```python
from build123d import *

# Parameters (mm, degrees)
F0_R      = 127
F1_DEPTH  = 254
F3_DEPTH  = 254
F4_DEPTH  = 25.4
F5_R      = 49.5787296889
F6_DEPTH  = 210.82
F7_R      = 54.002568176
F8_DEPTH  = 254
F9_R      = 52.4914497997
F10_DEPTH = 254


with BuildPart() as f1:
    # F0 (on Top) → F1 (new body)
    with BuildSketch(Plane.XY):
        Circle(F0_R)
    extrude(amount=F1_DEPTH)

    # F2 (on face) → F3 (join)
    with BuildSketch(Plane.XY.offset(254)):
        with BuildLine():
            Line((559.1962337494, 39.9803072214), (126.6766473602, 9.056876591))
            ThreePointArc((126.6766473602, 9.056876591), (126.9191360961, 4.5313234964), (127, 0))
            ThreePointArc((127, 0), (124.2007035095, -26.5176403124), (115.9262165711, -51.8662926332))
            Line((115.9262165711, -51.8662926332), (503.8578976831, -62.8307757108))
            Line((503.8578976831, -62.8307757108), (513.781719797, -288.9111098311))
            Line((513.781719797, -288.9111098311), (573.5178616361, -286.2889850555))
            Line((573.5178616361, -286.2889850555), (559.1962337494, 39.9803072214))
        make_face()
    extrude(amount=-F3_DEPTH)

    # F4 (add): a face of the model
    f4_faces = [f1.faces().sort_by_distance(p)[0] for p in [
        (309.8920571271, -57.348534172, 127),
    ]]
    extrude(f4_faces, amount=F4_DEPTH)

    # F5 (on face) → F6 (cut)
    with BuildSketch(Plane(origin=(-2.08986034, -73.9408350817, 0), x_dir=(0.9996008136, -0.0282526711, 0), z_dir=(-0.0282526711, -0.9996008136, 0))):
        with Locations((185.5181306601, 163.3890718222)):
            Circle(F5_R)
    extrude(amount=-F6_DEPTH, mode=Mode.SUBTRACT)

    # F7 (on face) → F8 (cut)
    with BuildSketch(Plane(origin=(-2.08986034, -73.9408350817, 0), x_dir=(0.9996008136, -0.0282526711, 0), z_dir=(-0.0282526711, -0.9996008136, 0))):
        with Locations((322.3161399364, 168.2878434658)):
            Circle(F7_R)
    extrude(amount=-F8_DEPTH, mode=Mode.SUBTRACT)

    # F9 (on face) → F10 (cut)
    with BuildSketch(Plane(origin=(-2.08986034, -73.9408350817, 0), x_dir=(0.9996008136, -0.0282526711, 0), z_dir=(-0.0282526711, -0.9996008136, 0))):
        with Locations((390.9286558628, 74.9529749155)):
            Circle(F9_R)
    extrude(amount=-F10_DEPTH, mode=Mode.SUBTRACT)


solid = f1.part
```
Design review of the part built by this model. Coordinates are the model's own, in mm. A direction names the side the tool comes from. Coordinates: 2 decimals unless noted, no trailing zeros. Loops run counter-clockwise (first coordinate to the right, second up) from the corner with the lowest first, then second, coordinate; pieces in that order, holes last. Notation, with made-up numbers: M 54.5,3.25 L 103.5,3.25 A19 cw 103.5,33.25 Z; hole C -35,-1 d6. An arc over 180 degrees is marked long. One line per question, with ' | ' between items.
(1) Draft analysis for pull direction X (two halves, no side actions). For faces 1 (the face through (230.49, -32.44, 144.4)), 2 (the face through (221, -33, 0)), 3 (the face through (543.23, -287.62, 128.78)), state which applies: released by +X, released by -X, zero draft, split by the parting line, or undercut.
Filled in:
face 1: undercut | face 2: zero draft | face 3: released by +X
(2) We need section B-B (y = -11.5). Count the separate pieces of the cut face and the enclosed holes in it, and give its area (3 significant figures).
Filled in:
separate pieces: 1 | enclosed holes: 3 | area: 149,000 mm^2
(3) Wall thickness on probe 1 along Z at (x, y) = (353, -18); probe 2 along X at (y, z) = (-3, 109); probe 3 along X at (y, z) = (-113, 118): over which ranges is each line inside the solid? List them lowest first.
Filled in:
probe 1: z = 0 to 38.29, 111.62 to 124.11, 212.47 to 254 | probe 2: x = -126.96 to 351.03, 430.97 to 561.08 | probe 3: x = -57.97 to 57.97, 506.06 to 565.91
(4) We need section A-A (z = 196). Give the boundary of the cut face in (x, y).
Filled in:
outline: M 115.21,-77.26 L 146.03,-78.13 L 148.53,10.62 L 126.68,9.06 A127 ccw long 115.93,-51.87 Z; M 220.68,-80.24 L 273.77,-81.74 L 276.64,19.78 L 223.4,15.97 Z; M 366.43,-84.36 L 503.14,-88.22 L 503.86,-62.83 L 513.78,-288.91 L 573.52,-286.29 L 559.2,39.98 L 369.56,26.42 Z
(5) Machinability: for faces 4 (the face through (371.517, -29.466, 147.605)), 5 (the face through (394.02, 28.17, 128.78)), 6 (the face through (566.457, -125.438, 128.778)), which of the approach directions +Z, -Z, +X, -X, +Y, -Y give a long, thin tool a straight path to every point of the face, cutting with its end or side? Answer none if there is none.
Filled in:
face 4: none | face 5: +Z, -Z, +Y | face 6: +Z, -Z, +X, +Y
(6) For pin 1 Ø1 at (x, z) = (262.5, 61.5) entering from -Y; pin 2 Ø1 at (y, z) = (35.5, 92.5) entering from +X; pin 3 Ø1 at (x, y) = (69.5, -35) entering from -Z; pin 4 Ø8 at (x, z) = (401, 203) entering from -Y, all flat-tipped, find the tip position at first contact; note any pin that passes through.
Filled in:
pin 1: stops at y = -81.43 | pin 2: stops at x = 559.41 | pin 3: stops at z = 0 | pin 4: stops at y = -85.45
(7) We need section D-D (y = -201). Give the boundary of the cut face in (x, z).
Filled in:
outline: M 509.92,0 L 569.77,0 L 569.77,254 L 509.92,254 Z
(8) We need section C-C (x = 0). Give the boundary of the cut face in (y, z), and give its area (3 significant figures).
Filled in:
outline: M -127,0 L 127,0 L 127,254 L -127,254 Z | area: 64,500 mm^2
